from build123d import *

# Parameters (mm, degrees)
SKETCH1_R           = 35
SKETCH1_R_2         = 19.685
SKETCH1_R_3         = 3.302
BOSS_EXTRUDE1_DEPTH = 9.271
SKETCH2_R           = 4.7625
CUT_EXTRUDE1_DEPTH  = 6.35


with BuildPart() as part:
    # Sketch1 → Boss-Extrude1 (new body)
    with BuildSketch(Plane(origin=(0, 0, 0), x_dir=(0, 0, -1), z_dir=(1, 0, 0))):
        Circle(SKETCH1_R)
        Circle(SKETCH1_R_2, mode=Mode.SUBTRACT)
        with Locations((0, 25.4)):
            Circle(SKETCH1_R_3, mode=Mode.SUBTRACT)
        with Locations((25.4, 0)):
            Circle(SKETCH1_R_3, mode=Mode.SUBTRACT)
        with Locations((0, -25.4)):
            Circle(SKETCH1_R_3, mode=Mode.SUBTRACT)
    extrude(amount=BOSS_EXTRUDE1_DEPTH)

    # Sketch2 → Cut-Extrude1 (cut)
    with BuildSketch(Plane.ZY):
        with Locations((0, 25.4)):
            Circle(SKETCH2_R)
        with Locations((0, -25.4)):
            Circle(SKETCH2_R)
        with Locations((-25.4, 0)):
            Circle(SKETCH2_R)
    extrude(amount=-CUT_EXTRUDE1_DEPTH, mode=Mode.SUBTRACT)


solid = part.part
Geometry: final body of the model. Coordinates: model frame, mm. A direction names the side the tool comes from. Coordinates: 2 decimals unless noted, no trailing zeros. Order: outer loops, then holes, each group sorted by start corner. A loop starts at its lowest first (then second) coordinate and runs counter-clockwise, first axis right, second up. Notation, with made-up numbers: M 67,6 L 76,6 A21 cw 76,25 Z; hole C 89,-14 d5. An arc over 180 degrees is marked long. One line per question, with ' | ' between items. Start each with the question number.
Item 1: Cut plane B-B, the plane z = -18. Return the cut outline in (x, y), then the cut area to 3 significant figures.
Item 2: Ray query, probe 1 along Y at (x, z) = (7, 0) (3 decimals); probe 2 along Y at (x, z) = (2, 0) (1 decimal); probe 3 along Z at (x, y) = (5, 3). Return the intervals inside material, ascending. Write a range as [from, to].
Item 3: Pin query (flat end, axial travel): pin 1 Ø1 at (x, y) = (7, 20.5) entering from -Z; pin 2 Ø5 at (y, z) = (-24, 2.5) entering from -X; pin 3 Ø7.5 at (y, z) = (-25.4, 0) entering from -X; pin 4 Ø1.5 at (x, y) = (6.5, -18.5) entering from +Z. Return the tip coordinate at first contact, or that it passes through.
Item 4: Cut plane A-A, the plane y = 0. Count the separate pieces of the cut face and the enclosed holes in it, then the cut area to 3 significant figures.
Item 5: Draft query along Z for faces 3 (the flat face through (9.271, -15, -15)), 4 (the cylindrical face through (5, -21, 28)), 5 (the flat face through (6.35, 1, -22)). Return one class per face: released by +Z, released by -Z, zero draft, split by the parting line, or undercut.
Item 6: Set-up query: faces 1 (the cylindrical face through (7.79, 28.674, 0.43)), 2 (the flat face through (6.35, 22, -1)). Return all of +Z, -Z, +X, -X, +Y, -Y with unobstructed straight access to the full face (end or side cutting, diameter ignored); none if empty.
Item 7: Cut plane C-C, the plane x = 7.75. Return the cut outline in (y, z) (3 decimals), then the cut area to 3 significant figures.
Item 8: Cut plane D-D, the plane y = 25.4. Return the cut outline in (x, z).
A:
1) outline: M 0,-30.02 L 9.27,-30.02 L 9.27,-7.97 L 0,-7.97 Z; M 0,7.97 L 9.27,7.97 L 9.27,30.02 L 0,30.02 Z | area: 409 mm2
2) probe 1: y = [-35, -28.702], [-22.098, -19.685], [19.685, 22.098], [28.702, 35] | probe 2: y = [-35, -30.2], [-20.6, -19.7], [19.7, 20.6], [30.2, 35] | probe 3: z = [-34.87, -29.1], [-21.7, -19.46], [19.46, 34.87]
3) pin 1: stops at z = -28.72 | pin 2: stops at x = 0 | pin 3: stops at x = 6.35 | pin 4: stops at z = 30.17
4) separate pieces: 3 | enclosed holes: 0 | area: 204 mm2
5) face 3: zero draft | face 4: split by the parting line | face 5: undercut
6) face 1: +X, -X | face 2: -X
7) outline: C 0,0 d70; hole C -25.4,0 d6.604; hole C 0,0 d39.37; hole C 0,-25.4 d6.604; hole C 25.4,0 d6.604 | area: 2,530 mm2
8) outline: M 0,-24.08 L 9.27,-24.08 L 9.27,-3.3 L 6.35,-3.3 L 6.35,-4.76 L 0,-4.76 Z; M 0,4.76 L 6.35,4.76 L 6.35,3.3 L 9.27,3.3 L 9.27,24.08 L 0,24.08 Z
